For this review, take the finished solid that the model builds, in its own axes (mm). A direction names the side the tool comes from. Give positions to 0.01 mm unless a question says otherwise; leave off trailing zeros. Loops run counter-clockwise (first coordinate to the right, second up) from the corner with the lowest first, then second, coordinate; pieces in that order, holes last. Notation, with made-up numbers: (82.5, 68.25) - (103.5, 68.25) arc R34 cw to (103.5, 107.25) - close; hole circle Ø3 at (83, 10). An arc over 180 degrees is marked (long way). Answer in a Markdown table with one row per item.
```python
from build123d import *

# Parameters (mm, degrees)
SKETCH1_W           = 66
SKETCH1_H           = 58.3
SKETCH1_R           = 2.75
BOSS_EXTRUDE1_DEPTH = 29
CUT_EXTRUDE1_START  = -29
CUT_EXTRUDE1_DEPTH  = 23.6
SKETCH4_R           = 11.5
CUT_EXTRUDE2_DEPTH  = 2.3
CUT_EXTRUDE3_REACH  = 54.723
SKETCH5_R           = 2.05
SKETCH6_W           = 10
SKETCH6_H           = 7.9
SKETCH6_R           = 2.05
BOSS_EXTRUDE2_DEPTH = 3
BOSS_EXTRUDE4_DEPTH = 7.9
BOSS_EXTRUDE5_START = -50.4
BOSS_EXTRUDE5_DEPTH = 7.9
CUT_EXTRUDE4_START  = -58.3
SKETCH8_R           = 4.05
CUT_EXTRUDE4_DEPTH  = 58.3
CUT_EXTRUDE5_REACH  = 80.031
SKETCH10_W          = 3
SKETCH10_H          = 6
SKETCH10_W_2        = 4.2
SKETCH10_W_3        = 0.4
SKETCH10_H_2        = 7.6
CUT_EXTRUDE6_REACH  = 84.74
SKETCH11_R          = 1.55


with BuildPart() as part:
    # Sketch1 → Boss-Extrude1 (new body)
    with BuildSketch(Plane(origin=(0, 0, 0), x_dir=(1, 0, 0), z_dir=(0, 1, 0))):
        Rectangle(SKETCH1_W, SKETCH1_H)
        with Locations(Location((-3.85, 0, 0), (0, 0, 90))):
            Circle(SKETCH1_R, mode=Mode.SUBTRACT)
    extrude(amount=BOSS_EXTRUDE1_DEPTH)

    # Sketch3 → Cut-Extrude1 (cut)
    with BuildSketch(Plane(origin=(0, 29, 0), x_dir=(1, 0, 0), z_dir=(0, 1, 0)).offset(CUT_EXTRUDE1_START)):
        Polygon((-33, 21.25), (-33, -21.25), (-25.1, -21.25), (-25.1, -29.15), (17.4, -29.15), (17.4, 29.15), (-25.1, 29.15), (-25.1, 21.25), align=None)
    extrude(amount=CUT_EXTRUDE1_DEPTH, mode=Mode.SUBTRACT)

    # Sketch4 → Cut-Extrude2 (cut)
    with BuildSketch(Plane.XZ.offset(-23.6)):
        with Locations(Location((-3.85, 0, 0), (0, 0, 270))):
            Circle(SKETCH4_R)
    extrude(amount=-CUT_EXTRUDE2_DEPTH, mode=Mode.SUBTRACT)

    # Sketch5 → Cut-Extrude3 (cut, up to next)
    with BuildSketch(Plane(origin=(0, 29, 0), x_dir=(1, 0, 0), z_dir=(0, 1, 0)), mode=Mode.PRIVATE) as cut_extrude3_sk1:
        with Locations(Location((-19.35, 15.5, 0), (0, 0, 270))):
            Circle(SKETCH5_R)
    cut_extrude3_tool1 = extrude(cut_extrude3_sk1.sketch, amount=-CUT_EXTRUDE3_REACH, mode=Mode.PRIVATE) & part.part
    # Sketch5 → Cut-Extrude3 (cut, up to next)
    with BuildSketch(Plane(origin=(0, 29, 0), x_dir=(1, 0, 0), z_dir=(0, 1, 0)), mode=Mode.PRIVATE) as cut_extrude3_sk2:
        with Locations(Location((11.65, 15.5, 0), (0, 0, 90))):
            Circle(SKETCH5_R)
    cut_extrude3_tool2 = extrude(cut_extrude3_sk2.sketch, amount=-CUT_EXTRUDE3_REACH, mode=Mode.PRIVATE) & part.part
    # Sketch5 → Cut-Extrude3 (cut, up to next)
    with BuildSketch(Plane(origin=(0, 29, 0), x_dir=(1, 0, 0), z_dir=(0, 1, 0)), mode=Mode.PRIVATE) as cut_extrude3_sk3:
        with Locations(Location((11.65, -15.5, 0), (0, 0, 270))):
            Circle(SKETCH5_R)
    cut_extrude3_tool3 = extrude(cut_extrude3_sk3.sketch, amount=-CUT_EXTRUDE3_REACH, mode=Mode.PRIVATE) & part.part
    # Sketch5 → Cut-Extrude3 (cut, up to next)
    with BuildSketch(Plane(origin=(0, 29, 0), x_dir=(1, 0, 0), z_dir=(0, 1, 0)), mode=Mode.PRIVATE) as cut_extrude3_sk4:
        with Locations(Location((-19.35, -15.5, 0), (0, 0, 90))):
            Circle(SKETCH5_R)
    cut_extrude3_tool4 = extrude(cut_extrude3_sk4.sketch, amount=-CUT_EXTRUDE3_REACH, mode=Mode.PRIVATE) & part.part
    add(cut_extrude3_tool1.solids().sort_by_distance((-19.35, 29, -15.5))[0], mode=Mode.SUBTRACT)
    add(cut_extrude3_tool2.solids().sort_by_distance((11.65, 29, -15.5))[0], mode=Mode.SUBTRACT)
    add(cut_extrude3_tool3.solids().sort_by_distance((11.65, 29, 15.5))[0], mode=Mode.SUBTRACT)
    add(cut_extrude3_tool4.solids().sort_by_distance((-19.35, 29, 15.5))[0], mode=Mode.SUBTRACT)

    # Sketch6 → Boss-Extrude2 (add)
    # profile 1 of 4: a face of its own
    with BuildSketch(Plane.XZ):
        with Locations((-38, 25.2)):
            Rectangle(SKETCH6_W, SKETCH6_H)
        with Locations(Location((-39.3, 25.2, 0), (0, 0, 270))):
            Circle(SKETCH6_R, mode=Mode.SUBTRACT)
    # profile 2 of 4: a face of its own
    with BuildSketch(Plane.XZ):
        with Locations((-38, -25.2)):
            Rectangle(SKETCH6_W, SKETCH6_H)
        with Locations(Location((-39.3, -25.2, 0), (0, 0, 270))):
            Circle(SKETCH6_R, mode=Mode.SUBTRACT)
    # profile 3 of 4: a face of its own
    with BuildSketch(Plane.XZ):
        with Locations((38, 25.2)):
            Rectangle(SKETCH6_W, SKETCH6_H)
        with Locations(Location((39.3, 25.2, 0), (0, 0, 270))):
            Circle(SKETCH6_R, mode=Mode.SUBTRACT)
    # profile 4 of 4: a face of its own
    with BuildSketch(Plane.XZ):
        with Locations((38, -25.2)):
            Rectangle(SKETCH6_W, SKETCH6_H)
        with Locations(Location((39.3, -25.2, 0), (0, 0, 270))):
            Circle(SKETCH6_R, mode=Mode.SUBTRACT)
    extrude(amount=-BOSS_EXTRUDE2_DEPTH)

    # Sketch7 → Boss-Extrude4 (add)
    with BuildSketch(Plane(origin=(0, 0, -29.15), x_dir=(-1, 0, 0), z_dir=(0, 0, -1))):
        with BuildLine():
            ThreePointArc((35.5, 3), (33.732233047, 3.732233047), (33, 5.5))
            Line((33, 5.5), (33, 3))
            Line((33, 3), (35.5, 3))
        make_face()
        with BuildLine():
            ThreePointArc((-33, 6), (-33.878679656, 3.878679656), (-36, 3))
            Line((-36, 3), (-33, 3))
            Line((-33, 3), (-33, 6))
        make_face()
    extrude(amount=-BOSS_EXTRUDE4_DEPTH)

    # Sketch7<5> → Boss-Extrude5 (add)
    with BuildSketch(Plane(origin=(0, 0, -29.15), x_dir=(-1, 0, 0), z_dir=(0, 0, -1)).offset(BOSS_EXTRUDE5_START)):
        with BuildLine():
            ThreePointArc((35.5, 3), (33.732233047, 3.732233047), (33, 5.5))
            Line((33, 5.5), (33, 3))
            Line((33, 3), (35.5, 3))
        make_face()
        with BuildLine():
            ThreePointArc((-33, 6), (-33.878679656, 3.878679656), (-36, 3))
            Line((-36, 3), (-33, 3))
            Line((-33, 3), (-33, 6))
        make_face()
    extrude(amount=-BOSS_EXTRUDE5_DEPTH)

    # Sketch8 → Cut-Extrude4 (cut)
    with BuildSketch(Plane.XY.offset(29.15).offset(CUT_EXTRUDE4_START)):
        with Locations(Location((26.05, 18, 0), (0, 0, 180))):
            Circle(SKETCH8_R)
    extrude(amount=CUT_EXTRUDE4_DEPTH, mode=Mode.SUBTRACT)

    # Sketch10 → Cut-Extrude5 (cut, up to next)
    with BuildSketch(Plane(origin=(0, 0, -29.15), x_dir=(-1, 0, 0), z_dir=(0, 0, -1)), mode=Mode.PRIVATE) as cut_extrude5_sk1:
        with Locations((-21.8, 26)):
            Rectangle(SKETCH10_W, SKETCH10_H)
    cut_extrude5_tool1 = extrude(cut_extrude5_sk1.sketch, amount=-CUT_EXTRUDE5_REACH, mode=Mode.PRIVATE) & part.part
    # Sketch10 → Cut-Extrude5 (cut, up to next)
    with BuildSketch(Plane(origin=(0, 0, -29.15), x_dir=(-1, 0, 0), z_dir=(0, 0, -1)), mode=Mode.PRIVATE) as cut_extrude5_sk2:
        with Locations((-30.9, 26)):
            Rectangle(SKETCH10_W_2, SKETCH10_H)
    cut_extrude5_tool2 = extrude(cut_extrude5_sk2.sketch, amount=-CUT_EXTRUDE5_REACH, mode=Mode.PRIVATE) & part.part
    # Sketch10 → Cut-Extrude5 (cut, up to next)
    with BuildSketch(Plane(origin=(0, 0, -29.15), x_dir=(-1, 0, 0), z_dir=(0, 0, -1)), mode=Mode.PRIVATE) as cut_extrude5_sk3:
        with Locations((-26.05, 25.2)):
            Rectangle(SKETCH10_W_3, SKETCH10_H_2)
    cut_extrude5_tool3 = extrude(cut_extrude5_sk3.sketch, amount=-CUT_EXTRUDE5_REACH, mode=Mode.PRIVATE) & part.part
    add(cut_extrude5_tool1.solids().sort_by_distance((21.8, 26, -29.15))[0], mode=Mode.SUBTRACT)
    add(cut_extrude5_tool2.solids().sort_by_distance((30.9, 26, -29.15))[0], mode=Mode.SUBTRACT)
    add(cut_extrude5_tool3.solids().sort_by_distance((26.05, 25.2, -29.15))[0], mode=Mode.SUBTRACT)

    # Cut-Extrude6: up to this face of the body (flat: up to its plane)
    cut_extrude6_end = Plane(part.part.faces().sort_by_distance((23.3, 26, 0))[0])
    # Sketch11 → Cut-Extrude6 (cut, up to the picked face)
    with BuildSketch(Plane(origin=(28.8, 0, 0), x_dir=(0, 0, -1), z_dir=(1, 0, 0)), mode=Mode.PRIVATE) as cut_extrude6_sk1:
        with Locations((-21.15, 25.6)):
            Circle(SKETCH11_R)
    cut_extrude6_tool1 = split(extrude(cut_extrude6_sk1.sketch, amount=-CUT_EXTRUDE6_REACH, mode=Mode.PRIVATE), bisect_by=cut_extrude6_end, keep=Keep.BOTH, mode=Mode.PRIVATE)
    # Sketch11 → Cut-Extrude6 (cut, up to the picked face)
    with BuildSketch(Plane(origin=(28.8, 0, 0), x_dir=(0, 0, -1), z_dir=(1, 0, 0)), mode=Mode.PRIVATE) as cut_extrude6_sk2:
        with Locations((21.15, 25.6)):
            Circle(SKETCH11_R)
    cut_extrude6_tool2 = split(extrude(cut_extrude6_sk2.sketch, amount=-CUT_EXTRUDE6_REACH, mode=Mode.PRIVATE), bisect_by=cut_extrude6_end, keep=Keep.BOTH, mode=Mode.PRIVATE)
    add(cut_extrude6_tool1.solids().sort_by(Axis((28.8, 25.6, 21.15), (-1, 0, 0)))[0], mode=Mode.SUBTRACT)
    add(cut_extrude6_tool2.solids().sort_by(Axis((28.8, 25.6, -21.15), (-1, 0, 0)))[0], mode=Mode.SUBTRACT)


solid = part.part
```
1. Wall thickness on line 1 (X direction, y = 27.1, z = 15.5); line 2 (X direction, y = 24.3, z = 0); line 3 (X direction, y = 27.7, z = 0): over which ranges is each line inside the solid? List them lowest first. Write a range as [from, to].
Values:
| item | result |
|---|---|
| line 1 | x = [-33, -21.4], [-17.3, 9.6], [13.7, 20.3], [23.3, 25.85], [26.25, 28.8] |
| line 2 | x = [-33, -15.35], [7.65, 20.3], [23.3, 25.85], [26.25, 28.8] |
| line 3 | x = [-33, -6.6], [-1.1, 20.3], [23.3, 25.85], [26.25, 28.8] |
2. Mouldability with a two-part tool opening along Y and no side actions: class faces 5 (the face through (22, 23, 0)), 6 (the face through (-39.21, 1.48, 27.25)), 7 (the face through (27, 0, 0)), 8 (the face through (27.543, 25.006, -22.582)) as released by +Y, released by -Y, zero draft, split by the parting line, or undercut.
Values:
| item | result |
|---|---|
| face 5 | released by +Y |
| face 6 | zero draft |
| face 7 | released by -Y |
| face 8 | undercut |
3. For faces 1 (the face through (-25.1, 12, -25)), 2 (the face through (42, 3, 25)), 3 (the face through (27.543, 25.006, 19.718)), 4 (the face through (-30, 12, 21.25)), list the 3-axis set-ups (+Z, -Z, +X, -X, +Y, -Y) from which the entire face can be reached by the end or side of a thin tool; tool diameter is ignored.
Values:
| item | result |
|---|---|
| face 1 | +Z, -Z, -Y |
| face 2 | +Z, -Z, +X, +Y |
| face 3 | +X |
| face 4 | -X, -Y |
4. We need section A-A, the plane z = 25.2. Count the separate pieces of the cut face and the enclosed holes in it, and give its area (3 significant figures).
Values:
| item | result |
|---|---|
| separate pieces | 3 |
| enclosed holes | 0 |
| area | 852 mm^2 |
5. We need section C-C, the plane z = 0. Give the boundary of the cut face in (x, y).
Values:
| item | result |
|---|---|
| outline | (-33, 23.6) - (-15.35, 23.6) - (-15.35, 25.9) - (-6.6, 25.9) - (-6.6, 29) - (-33, 29) - close; (-1.1, 25.9) - (7.65, 25.9) - (7.65, 23.6) - (17.4, 23.6) - (17.4, 0) - (33, 0) - (33, 23) - (28.8, 23) - (28.8, 29) - (26.25, 29) - (26.25, 22.05) arc R4.05 cw (long way) to (25.85, 22.05) - (25.85, 29) - (23.3, 29) - (23.3, 23) - (20.3, 23) - (20.3, 29) - (-1.1, 29) - close |
6. Clearance check with flat-ended pins moving along their axes: pin 1 (1.8 mm diameter, centred on x = 39, y = 4, fed in from -Z); pin 2 (12 mm diameter, centred on y = 25, z = 4.5, fed in from -X); pin 3 (2 mm diameter, centred on x = -38, z = 25.5, fed in from +Y); pin 4 (2.5 mm diameter, centred on x = 22, z = 7.5, fed in from +Y). State where each tip first meets the part, or that it passes through.
Values:
| item | result |
|---|---|
| pin 1 | passes through |
| pin 2 | stops at x = -33 |
| pin 3 | stops at y = 3 |
| pin 4 | stops at y = 23 |
7. We need section D-D, the plane y = 20.75. Give the boundary of the cut face in (x, z).
Values:
| item | result |
|---|---|
| outline | (-33, -29.15) - (-25.1, -29.15) - (-25.1, -21.25) - (-33, -21.25) - close; (-33, 21.25) - (-25.1, 21.25) - (-25.1, 29.15) - (-33, 29.15) - close; (17.4, -29.15) - (23.08, -29.15) - (23.08, 29.15) - (17.4, 29.15) - close; (29.02, -29.15) - (33, -29.15) - (33, 29.15) - (29.02, 29.15) - close |
8. We need section B-B, the plane x = -19.35. Give the boundary of the cut face in (y, z).
Values:
| item | result |
|---|---|
| outline | (23.6, -29.15) - (29, -29.15) - (29, -17.55) - (23.6, -17.55) - close; (23.6, -13.45) - (29, -13.45) - (29, 13.45) - (23.6, 13.45) - close; (23.6, 17.55) - (29, 17.55) - (29, 29.15) - (23.6, 29.15) - close |
